from build123d import *

# Parameters (mm, degrees)
BOSS_EXTRUDE1_DEPTH = 3
CUT_EXTRUDE1_DEPTH  = 103.574363269
CUT_EXTRUDE3_DEPTH  = 103.574363269
CUT_EXTRUDE4_DEPTH  = 103.574363269
SKETCH6_W           = 68.4
SKETCH6_H           = 3
CUT_EXTRUDE5_DEPTH  = 103.574363269
SKETCH7_R           = 5
CUT_EXTRUDE6_DEPTH  = 103.574363269
SKETCH11_R          = 5
CUT_EXTRUDE10_DEPTH = 103.574363269


with BuildPart() as part:
    # Sketch1 → Boss-Extrude1 (new body)
    with BuildSketch(Plane(origin=(0, 0, 0), x_dir=(1, 0, 0), z_dir=(0, 1, 0))):
        with BuildLine():
            Line((-30.029977361, -64.812867647), (30.029977361, -64.812867647))
            ThreePointArc((30.029977361, -64.812867647), (32.509837414, -64.500503794), (34.834773739, -63.582926471))
            ThreePointArc((34.834773739, -63.582926471), (0, 72.5), (-34.834773739, -63.582926471))
            ThreePointArc((-34.834773739, -63.582926471), (-32.509837414, -64.500503794), (-30.029977361, -64.812867647))
        make_face()
    extrude(amount=BOSS_EXTRUDE1_DEPTH)

    # Sketch2 → Cut-Extrude1 (cut, through all)
    with BuildSketch(Plane(origin=(0, 3, 0), x_dir=(1, 0, 0), z_dir=(0, 1, 0))):
        Polygon((-22.2, -49.675685802), (-22.2, -38), (22.2, -38), (22.2, -49.675685802), (34.2, -49.675685802), (34.2, 49.675685802), (22.2, 49.675685802), (22.2, 44), (-22.2, 44), (-22.2, 49.675685802), (-34.2, 49.675685802), (-34.2, -49.675685802), align=None)
    extrude(amount=-CUT_EXTRUDE1_DEPTH, mode=Mode.SUBTRACT)

    # Sketch4 → Cut-Extrude3 (cut, through all)
    with BuildSketch(Plane(origin=(0, 3, 0), x_dir=(1, 0, 0), z_dir=(0, 1, 0))):
        Polygon((-21.070156074, -50.026174921), (-0.648164763, -51.812867647), (-0.5, -50.11933666), (-20.921991311, -48.332643934), align=None)
        Polygon((21.070156074, -50.026174921), (20.921991311, -48.332643934), (0.5, -50.11933666), (0.648164763, -51.812867647), align=None)
    extrude(amount=-CUT_EXTRUDE3_DEPTH, mode=Mode.SUBTRACT)

    # Sketch5 → Cut-Extrude4 (cut, through all)
    with BuildSketch(Plane(origin=(0, 3, 0), x_dir=(1, 0, 0), z_dir=(0, 1, 0))):
        with BuildLine():
            Line((5.878186928, -51.355299998), (15.840133909, -50.48374257))
            Line((15.840133909, -50.48374257), (16.798847079, -61.441884249))
            ThreePointArc((16.798847079, -61.441884249), (16.568696824, -62.171827602), (15.889808123, -62.52523469))
            Line((15.889808123, -62.52523469), (7.920250539, -63.222480632))
            ThreePointArc((7.920250539, -63.222480632), (7.190307186, -62.992330377), (6.836900098, -62.313441677))
            Line((6.836900098, -62.313441677), (5.878186928, -51.355299998))
        make_face()
        Polygon((16.688163844, -48.703055841), (4.733827467, -49.748924754), (4.559515981, -47.756535357), (16.513852358, -46.710666444), align=None)
        Polygon((-16.513852358, -46.710666444), (-4.559515981, -47.756535357), (-4.733827467, -49.748924754), (-16.688163844, -48.703055841), align=None)
        with BuildLine():
            Line((-7.920250539, -63.222480632), (-15.889808123, -62.52523469))
            ThreePointArc((-15.889808123, -62.52523469), (-16.568696824, -62.171827602), (-16.798847079, -61.441884249))
            Line((-16.798847079, -61.441884249), (-15.840133909, -50.48374257))
            Line((-15.840133909, -50.48374257), (-5.878186928, -51.355299998))
            Line((-5.878186928, -51.355299998), (-6.836900098, -62.313441677))
            ThreePointArc((-6.836900098, -62.313441677), (-7.190307186, -62.992330377), (-7.920250539, -63.222480632))
        make_face()
    extrude(amount=-CUT_EXTRUDE4_DEPTH, mode=Mode.SUBTRACT)

    # Sketch6 → Cut-Extrude5 (cut, through all)
    with BuildSketch(Plane(origin=(0, 3, 0), x_dir=(1, 0, 0), z_dir=(0, 1, 0))):
        with Locations((0, 51.175685802)):
            Rectangle(SKETCH6_W, SKETCH6_H)
    extrude(amount=-CUT_EXTRUDE5_DEPTH, mode=Mode.SUBTRACT)


with BuildPart() as cut_extrude5_kept_piece:
    # of the separate pieces the step leaves, the one the design keeps (cut_extrude5_pieces_kept)
    add(part.part.solids().sort_by_distance((-34.834773739, 0, 63.582926471))[0])

    # Sketch7 → Cut-Extrude6 (cut, through all)
    with BuildSketch(Plane(origin=(0, 3, 0), x_dir=(1, 0, 0), z_dir=(0, 1, 0))):
        with Locations(Location((-30, -57, 0), (0, 0, 270))):
            Circle(SKETCH7_R)
        with Locations(Location((30, -57, 0), (0, 0, 270))):
            Circle(SKETCH7_R)
    extrude(amount=-CUT_EXTRUDE6_DEPTH, mode=Mode.SUBTRACT)

    # Sketch11 → Cut-Extrude10 (cut, through all)
    with BuildSketch(Plane(origin=(0, 3, 0), x_dir=(1, 0, 0), z_dir=(0, 1, 0))):
        with Locations(Location((0, 65, 0), (0, 0, 270))):
            Circle(SKETCH11_R)
    extrude(amount=-CUT_EXTRUDE10_DEPTH, mode=Mode.SUBTRACT)


solid = cut_extrude5_kept_piece.part
Build history of the part. All positions in model axes, mm. A direction names the side the tool comes from. Give positions to 0.01 mm unless a question says otherwise; leave off trailing zeros. Order: outer loops, then holes, each group sorted by start corner. A loop starts at its lowest first (then second) coordinate and runs counter-clockwise, first axis right, second up. Notation, with made-up numbers: M 50.5,6 L 72.5,6 A21 cw 72.5,30 Z; hole C -14,52 d7. An arc over 180 degrees is marked long. Use one line per item in the form item = value.
Q1. Which spindle directions (+Z, -Z, +X, -X, +Y, -Y) get a long thin tool onto all of the face, cutting with end or side? Do faces 1 (the cylindrical face through (32.48, 1.48, 64.51)), 2 (the flat face through (-3.3, 1.52, 51.58)). Say none if no direction does.
Conclusion:
face_1 = +Z, +X, +Y, -Y
face_2 = +Y, -Y
Q2. Pull direction X, two halves, no side cores. Call faces 3 (the cylindrical face through (-32.544, 1.479, 64.492)), 4 (the flat face through (16.313, 1.521, 55.886)), 5 (the flat face through (37, 3, 1)), 6 (the flat face through (-34.2, 2, -1)): released by +X, released by -X, zero draft, split by the parting line, or undercut.
Conclusion:
face_3 = released by -X
face_4 = undercut
face_5 = zero draft
face_6 = undercut
Q3. Pin check, flat tips, straight feed: P1, Ø1.5, axis at y = 2, z = 21.5, coming from the +X side; P2, Ø0.9, axis at x = 28.5, y = 1, coming from the -Z side. Stop position of each tip, or through.
Conclusion:
P1 = 69.47
P2 = -66.85
Q4. Wall check: probe 1 along Z at (x, y) = (-14, 0.3); probe 2 along X at (y, z) = (1.7, 57); probe 3 along Z at (x, y) = (4, 1.6). Give the ranges that are in metal, low to high.
Conclusion:
probe_1 = -71.14 to -52.68, 38 to 46.93, 62.69 to 64.81
probe_2 = -44.8 to -35, -25 to -16.41, -6.37 to 6.37, 16.41 to 25, 35 to 44.8
probe_3 = -72.39 to -68, -62 to -52.68, 38 to 49.81, 51.52 to 64.81
Q5. Slice it at C-C, the plane y = 0.6. State how many separate pieces and enclosed holes the cut face has, and give its area (3 significant figures).
Conclusion:
separate_pieces = 1
enclosed_holes = 6
area = 9,100 mm2
Q6. Slice it at D-D, the plane z = 26. Write the cut outline in (x, y), and give its area (3 significant figures).
Conclusion:
outline = M -67.68,0 L -34.2,0 L -34.2,3 L -67.68,3 Z; M 34.2,0 L 67.68,0 L 67.68,3 L 34.2,3 Z
area = 201 mm2
Q7. Slice it at B-B, the plane x = 12. Write the cut outline in (y, z), and give its area (3 significant figures).
Conclusion:
outline = M 0,-71.5 L 3,-71.5 L 3,-52.68 L 0,-52.68 Z; M 0,38 L 3,38 L 3,47.11 L 0,47.11 Z; M 0,62.87 L 3,62.87 L 3,64.81 L 0,64.81 Z
area = 89.6 mm2
Q8. Slice it at A-A, the plane z = 0. Write the cut outline in (x, y).
Conclusion:
outline = M -72.5,0 L -34.2,0 L -34.2,3 L -72.5,3 Z; M 34.2,0 L 72.5,0 L 72.5,3 L 34.2,3 Z
